Check sheet for the drawn part. Datum: minimum x, y, z corner. Units: mm. A direction names the side the tool comes from. Round coordinates to 2 decimals unless told otherwise and drop trailing zeros. Write each loop counter-clockwise with the first axis right and the second up, starting at its lowest first coordinate (ties: lowest second). Pieces come first, ordered by that corner, then holes.
Item 1: Cross-section at C-C on z = 12. Enter the section's corners in (x, y).
Item 2: Material ranges on line 1 (Y direction, x = 10.5, z = 1.65); line 2 (Z direction, x = 6, y = 0.7); line 3 (Y direction, x = 20, z = 1.55), recorded low to high.
Item 3: Cross-section at D-D on y = 16.5. Enter the section's corners in (x, z).
Item 4: Go/stop test with flat-tipped pins: pin 1 Ø1.5 at (x, z) = (29.5, 4) entering from +Y; pin 2 Ø6 at (x, y) = (26.5, 9) entering from +Z. Record where each tip stops, or that it passes through.
Item 5: Cross-section at B-B on x = 34. Enter the section's corners in (y, z).
Item 6: Tool access check on the marked faces 1 and 2. Record the directions out of +Z, -Z, +X, -X, +Y, -Y that give a thin tool (end or side, any length) a straight path to the whole face; none if there is none.
Item 7: Cross-section at A-A on y = 13.5. Enter the section's corners in (x, z).
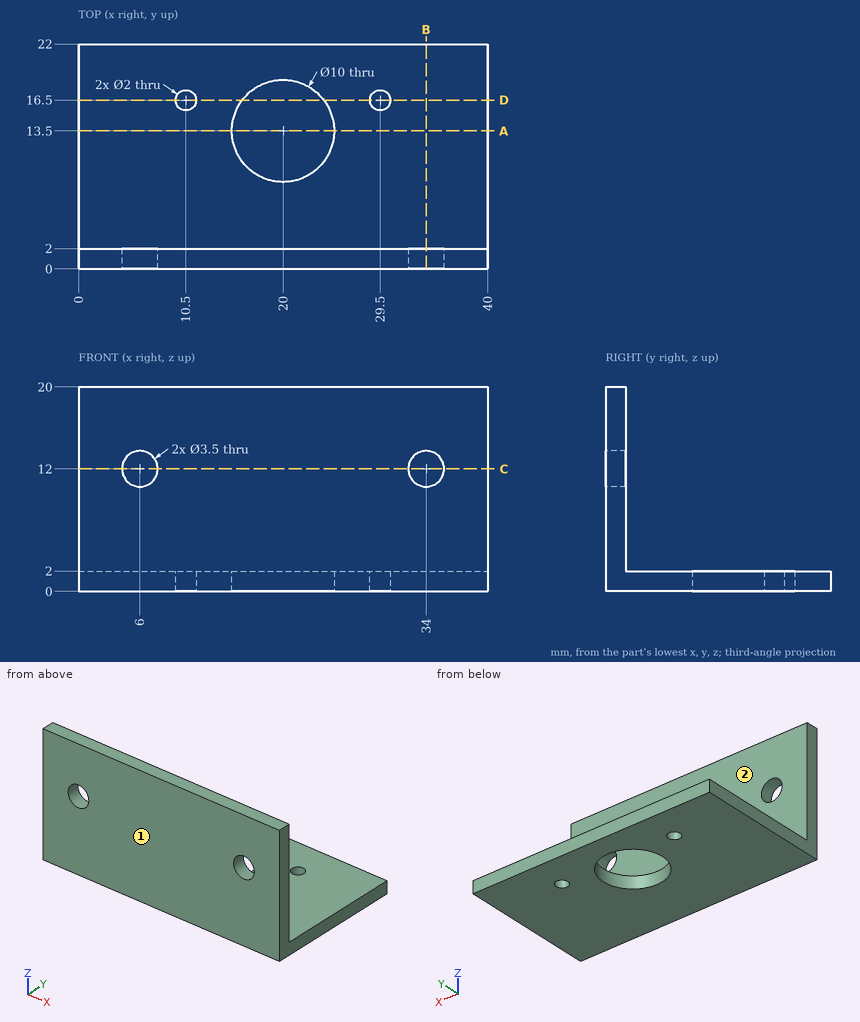
Response values:
1. outline: (0, 0) - (4.25, 0) - (4.25, 2) - (0, 2) - close; (7.75, 0) - (32.25, 0) - (32.25, 2) - (7.75, 2) - close; (35.75, 0) - (40, 0) - (40, 2) - (35.75, 2) - close
2. line 1: y = 0 to 15.5, 17.5 to 22
2. line 2: z = 0 to 10.25, 13.75 to 20
2. line 3: y = 0 to 8.5, 18.5 to 22
3. outline: (0, 0) - (9.5, 0) - (9.5, 2) - (0, 2) - close; (11.5, 0) - (16, 0) - (16, 2) - (11.5, 2) - close; (24, 0) - (28.5, 0) - (28.5, 2) - (24, 2) - close; (30.5, 0) - (40, 0) - (40, 2) - (30.5, 2) - close
4. pin 1: stops at y = 2
4. pin 2: stops at z = 2
5. outline: (0, 0) - (22, 0) - (22, 2) - (2, 2) - (2, 10.25) - (0, 10.25) - close; (0, 13.75) - (2, 13.75) - (2, 20) - (0, 20) - close
6. face 1: +Z, -Z, +X, -X, -Y
6. face 2: +Z, +X, -X, +Y
7. outline: (0, 0) - (15, 0) - (15, 2) - (0, 2) - close; (25, 0) - (40, 0) - (40, 2) - (25, 2) - close
